Check sheet for the modelled part. Datum: model origin and axes. Units: mm. Coordinates: 2 decimals unless noted, no trailing zeros. Write each loop counter-clockwise with the first axis right and the second up, starting at its lowest first coordinate (ties: lowest second). Pieces come first, ordered by that corner, then holes. Notation, with made-up numbers: (-39.75, 43) - (8.25, 43) arc R12 cw to (8.25, 60) - close; hole circle Ø9 at (61.25, 6.5). An arc over 180 degrees is marked (long way). Write each question's results on one line, items separated by ' | '.
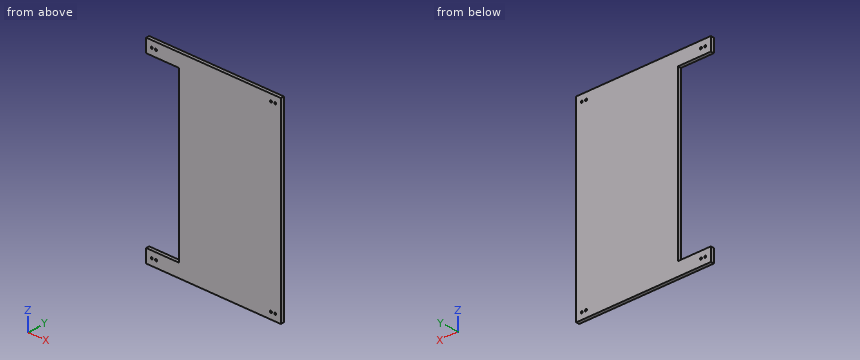
Autodesk Inventor part; units mm, degrees
ref_plane "YZ Plane" through (0, 0, 0) normal (1, 0, 0) x (0, 1, 0)
ref_plane "XZ Plane" through (0, 0, 0) normal (0, 1, 0) x (-1, 0, 0)
ref_plane "XY Plane" through (0, 0, 0) normal (0, 0, 1) x (1, 0, 0)
sketch "Esquisse1" plane through (0, 0, 0) normal (0, 1, 0) x (-1, 0, 0)
  line L0 (138.2405, 132.2434) -> (-66.7595, 132.2434)
  line L1 (-66.7595, 132.2434) -> (-66.7595, -157.7566)
  line L2 (-66.7595, -157.7566) -> (138.2405, -157.7566)
  line L3 (138.2405, -157.7566) -> (138.2405, 132.2434)
  point P0 (0, 0)
  dimension "d0" = 290
  dimension "d1" = 205
extrude "Extrusion1" add sketch "Esquisse1" along normal blind 5
sketch "Esquisse2" plane through (0, 5, 0) normal (0, 1, 0) x (1, 0, 0)
  line L0 (-138.2405, 157.7566) -> (-138.2405, -132.2434)
  line L1 (-138.2405, -112.2434) -> (-88.2405, -112.2434)
  line L2 (-88.2405, -112.2434) -> (-88.2405, 137.7566)
  line L3 (-88.2405, 137.7566) -> (-138.2405, 137.7566)
  line L4 (-138.2405, 137.7566) -> (-138.2405, -112.2434)
  line L5 (-138.2405, -132.2434) -> (66.7595, -132.2434)
  line L6 (66.7595, 157.7566) -> (-138.2405, 157.7566)
  point P0 (0, 0)
  dimension "d4" = 20
  dimension "d5" = 20
  dimension "d6" = 50
extrude "Extrusion2" cut sketch "Esquisse2" against normal up to next
sketch "Esquisse3" plane through (0, 5, 0) normal (0, 1, 0) x (1, 0, 0)
  circle A0 centre (58.2595, 147.7566) radius 1.5
  circle A1 centre (51.7595, 147.7566) radius 1.5
  circle A2 centre (58.2595, -122.2434) radius 1.5
  circle A3 centre (51.7595, -122.2434) radius 1.5
  circle A4 centre (-123.2405, -122.2434) radius 1.5
  circle A5 centre (-129.7405, -122.2434) radius 1.5
  circle A6 centre (-123.2405, 147.7566) radius 1.5
  circle A7 centre (-129.7405, 147.7566) radius 1.5
  point P0 (0, 0)
extrude "Extrusion3" cut sketch "Esquisse3" against normal up to next
properties part number "étage"
1. Sectioned sample at B-B (y = 2.5). Give the number of separate pieces and of enclosed holes in the cut face, then the cut area to 3 significant figures.
Values follow:
separate pieces: 1 | enclosed holes: 8 | area: 46,900 mm^2
2. Sectioned sample at C-C (z = 102). Record the cut outline in (x, y).
Values follow:
outline: (-88.24, 0) - (66.76, 0) - (66.76, 5) - (-88.24, 5) - close
3. Go/stop test with flat-tipped pins: pin 1 (1.8 mm diameter, centred on x = 58.26, z = 122.24, fed in from -Y); pin 2 (2.5 mm diameter, centred on y = 2.5, z = 41, fed in from -X). Record where each tip stops, or that it passes through.
Values follow:
pin 1: passes through | pin 2: stops at x = -88.24
4. Sectioned sample at A-A (x = -102). Record the cut outline in (y, z).
Values follow:
outline: (0, -157.76) - (5, -157.76) - (5, -137.76) - (0, -137.76) - close; (0, 112.24) - (5, 112.24) - (5, 132.24) - (0, 132.24) - close
5. Material ranges on L1, parallel to Z at x = -104.5, y = 4.4; L2, parallel to Z at x = 53, y = 0.4; L3, parallel to X at y = 2.85, z = -86.5, recorded low to high. Write a range as [from, to].
Values follow:
L1: z = [-157.76, -137.76], [112.24, 132.24] | L2: z = [-157.76, -148.6], [-146.91, 121.4], [123.09, 132.24] | L3: x = [-88.24, 66.76]
